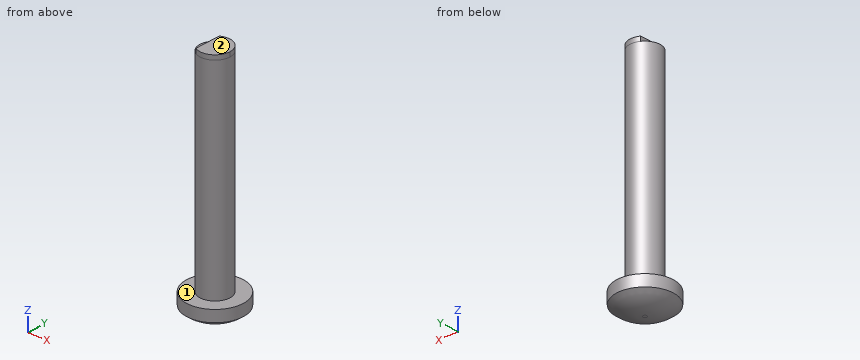
```python
from build123d import *

# Parameters (mm, degrees)
F0_W     = 1.27
F0_H     = 17.272
F3_DEPTH = 0.381


# Not quite as in the source:
# - a feature names something its author has since deleted; it is built from what else it names


with BuildPart() as f1:
    # F0 (on Front) → F1 (revolve)
    with BuildSketch(Plane.XZ):
        with Locations((-38.810752406, 44.918222718)):
            Rectangle(F0_W, F0_H)
        with BuildLine():
            Line((-38.175752406, 36.282222718), (-39.445752406, 36.282222718))
            Line((-39.445752406, 36.282222718), (-40.563352406, 36.282222718))
            Line((-40.563352406, 36.282222718), (-40.563352406, 35.9659250826))
            Line((-40.563352406, 35.9659250826), (-40.563352406, 35.329721868))
            ThreePointArc((-40.563352406, 35.329721868), (-39.5245363872, 34.7150900066), (-38.3366011083, 34.5012657344))
            Line((-38.3366011083, 34.5012657344), (-38.175752406, 34.5012657344))
            Line((-38.175752406, 34.5012657344), (-38.175752406, 35.1264222169))
            Line((-38.175752406, 35.1264222169), (-38.175752406, 36.282222718))
        make_face()
    revolve(axis=Axis((-38.175752406, 0, 44.918222718), (0, 0, -1)))

    # F2 (on face) → F3 (join)
    with BuildSketch(Plane.XY.offset(53.554222718)):
        with BuildLine():
            Line((-38.8069041073, 1.1020651206), (-38.8069041073, 0))
            Line((-38.8069041073, 0), (-38.8069041073, -1.1020651206))
            ThreePointArc((-38.8069041073, -1.1020651206), (-37.5388311631, -1.0987407931), (-36.905752406, 0))
            ThreePointArc((-36.905752406, 0), (-37.5388311631, 1.0987407931), (-38.8069041073, 1.1020651206))
        make_face()
    extrude(amount=F3_DEPTH)


solid = f1.part
```
Part model, mm, in its own coordinate system. Face numbers are marked on the shaded views. A direction names the side the tool comes from. Round coordinates to 2 decimals unless told otherwise and drop trailing zeros. Loops run counter-clockwise (first coordinate to the right, second up) from the corner with the lowest first, then second, coordinate; pieces in that order, holes last.
Item 1: Cut at A-A, the plane z = 49.5. Give the cut face in (x, y).
Item 2: 3-axis set-ups, long thin cutter, end or side, ignore diameter. For the marked faces 1 and 2: which of +Z, -Z, +X, -X, +Y, -Y reach the whole face in a straight line?
Item 3: Drill centre lines: line 1 (Y direction, x = -38.2, z = 49.25); line 2 (Y direction, x = -38.8, z = 45.5); line 3 (Z direction, x = -40.25, y = -0.7). Where is each one in solid material? Low to high.
A:
1. outline: circle Ø2.54 at (-38.18, 0)
2. face 1: +Z
2. face 2: +Z, +X, -X, +Y, -Y
3. line 1: y = -1.27 to 1.27
3. line 2: y = -1.11 to 1.11
3. line 3: z = 35.17 to 36.28
